The model under review builds one solid part; all positions refer to its coordinate system, in mm. A direction names the side the tool comes from. Round coordinates to 2 decimals unless told otherwise and drop trailing zeros. Order: outer loops, then holes, each group sorted by start corner. A loop starts at its lowest first (then second) coordinate and runs counter-clockwise, first axis right, second up.
1) Machinability: for faces 1 (the face through (-43, -12, -63)), 2 (the face through (27.5, 0, -7)), 3 (the face through (24.49, -20.6, 29.58)), 4 (the face through (24.54, 20.54, 29.58)), which of the approach directions +Z, -Z, +X, -X, +Y, -Y give a long, thin tool a straight path to every point of the face, cutting with its end or side? Answer none if there is none.
2) Consider section B-B (z = -100.25). Give the boundary of the cut face in (x, y), then the cut area to 3 significant figures.
3) Consider section D-D (x = 0). Give the boundary of the cut face in (y, z), then the cut area to 3 significant figures.
4) Mouldability with a two-part tool opening along Y and no side actions: class faces 5 (the face through (18.989, -22.576, 30.42)), 6 (the face through (16.04, 27.69, 29.58)), 7 (the face through (-38.7, -4.4, -3)) as pulls with the +Y half, pulls with the -Y half, needs draft (parallel to the pull), parting line crosses it, or undercut.
5) Consider section C-C (y = 0). Give the boundary of the cut face in (x, z).
6) To check wall thickness, follow L1, parallel to Y at x = 0, z = 59.1; L2, parallel to Y at x = 0, z = -78.25; L3, parallel to Z at x = 40, y = -11.4. State the ranges of each line that lie inside material, in increasing order.
7) Consider section A-A (x = -44.75). Give the boundary of the cut face in (y, z), then the cut area to 3 significant figures.
8) Clearance check with flat-ended pins moving along their axes: P1, Ø8, axis at y = 0, z = -6, coming from the +X side; P2, Ø2, axis at x = 34.5, y = -29.5, coming from the +Z side; P3, Ø0.5, axis at x = 42.5, y = -11.5, coming from the +Z side. State where each tip first meets the part, or that it passes through.
from build123d import *

# Parameters (mm, degrees)
CROQUIS1_R              = 32
SALIENTE_EXTRUIR1_DEPTH = 60
CROQUIS2_R              = 24.5
CORTAR_EXTRUIR1_DEPTH   = 2.5
CROQUIS3_W              = 5
CROQUIS3_H              = 5
CORTAR_EXTRUIR2_DEPTH   = 61
MATRIZC1_COUNT          = 18
CROQUIS4_R              = 26.25
SALIENTE_EXTRUIR2_DEPTH = 87.8
CROQUIS5_R              = 22.75
CORTAR_EXTRUIR3_DEPTH   = 37
SALIENTE_EXTRUIR3_REACH = 149.8
CROQUIS6_W              = 2.5
CROQUIS6_H              = 16
CROQUIS7_W              = 78
CROQUIS7_H              = 70
SALIENTE_EXTRUIR4_DEPTH = 61
CROQUIS8_W              = 10
CROQUIS8_H              = 1
SALIENTE_EXTRUIR5_DEPTH = 11.5
CROQUIS9_W              = 10
CROQUIS9_H              = 13
SALIENTE_EXTRUIR6_DEPTH = 1
CROQUIS10_W             = 11
CROQUIS10_H             = 10
SALIENTE_EXTRUIR7_DEPTH = 1
SALIENTE_EXTRUIR8_DEPTH = 1
CROQUIS12_R             = 2.5
CORTAR_EXTRUIR4_DEPTH   = 29
CROQUIS13_R             = 2.5
CORTAR_EXTRUIR5_DEPTH   = 1
CROQUIS14_R             = 2.5
CORTAR_EXTRUIR6_DEPTH   = 1
CROQUIS15_R             = 2.5
CORTAR_EXTRUIR7_DEPTH   = 1
CROQUIS16_R             = 3.5
SALIENTE_EXTRUIR9_DEPTH = 10


with BuildPart() as part:
    # Croquis1 → Saliente-Extruir1 (new body)
    with BuildSketch(Plane.XY):
        Circle(CROQUIS1_R)
    extrude(amount=SALIENTE_EXTRUIR1_DEPTH)

    # Croquis2 → Cortar-Extruir1 (cut)
    with BuildSketch(Plane.XY.offset(60)):
        Circle(CROQUIS2_R)
    extrude(amount=-CORTAR_EXTRUIR1_DEPTH, mode=Mode.SUBTRACT)

    # Croquis3 → Cortar-Extruir2 (cut, through all)
    with BuildSketch(Plane.XY.offset(60)):
        with Locations((0, 32)):
            Rectangle(CROQUIS3_W, CROQUIS3_H)
    cortar_extruir2 = extrude(amount=-CORTAR_EXTRUIR2_DEPTH, mode=Mode.SUBTRACT)

    # MatrizC1: Cortar-Extruir2 ×18 about axis
    matrizc1_axis = Axis((0, 0, 0), (0, 0, 1))
    for i in range(1, MATRIZC1_COUNT):
        add(cortar_extruir2.rotate(matrizc1_axis, i * 360 / MATRIZC1_COUNT), mode=Mode.SUBTRACT)

    # Croquis4 → Saliente-Extruir2 (add)
    with BuildSketch(Plane(origin=(0, 0, 0), x_dir=(-1, 0, 0), z_dir=(0, 0, -1))):
        Circle(CROQUIS4_R)
    extrude(amount=SALIENTE_EXTRUIR2_DEPTH)

    # Croquis5 → Cortar-Extruir3 (cut)
    with BuildSketch(Plane(origin=(0, 0, -87.8), x_dir=(-1, 0, 0), z_dir=(0, 0, -1))):
        Circle(CROQUIS5_R)
    extrude(amount=-CORTAR_EXTRUIR3_DEPTH, mode=Mode.SUBTRACT)

    # Croquis6 → Saliente-Extruir3 (add, up to next)
    with BuildSketch(Plane(origin=(0, 0, -87.8), x_dir=(-1, 0, 0), z_dir=(0, 0, -1)), mode=Mode.PRIVATE) as saliente_extruir3_sk1:
        with Locations((-26.25, 0)):
            Rectangle(CROQUIS6_W, CROQUIS6_H)
    saliente_extruir3_tool1 = extrude(saliente_extruir3_sk1.sketch, amount=-SALIENTE_EXTRUIR3_REACH, mode=Mode.PRIVATE) - part.part
    add(saliente_extruir3_tool1.solids().sort_by_distance((26.25, 0, -87.8))[0])

    # Croquis7 → Saliente-Extruir4 (add)
    with BuildSketch(Plane(origin=(0, 0, -13), x_dir=(-1, 0, 0), z_dir=(0, 0, -1))):
        Rectangle(CROQUIS7_W, CROQUIS7_H)
    extrude(amount=SALIENTE_EXTRUIR4_DEPTH)

    # Croquis8 → Saliente-Extruir5 (add)
    with BuildSketch(Plane.ZY.offset(39)):
        with Locations((-64.8, -11.5)):
            Rectangle(CROQUIS8_W, CROQUIS8_H)
        with Locations((-8, -7.5)):
            Rectangle(CROQUIS8_W, CROQUIS8_H)
    extrude(amount=SALIENTE_EXTRUIR5_DEPTH)

    # Croquis9 → Saliente-Extruir6 (add)
    with BuildSketch(Plane.ZY.offset(39)):
        with Locations((-8, -1.5)):
            Rectangle(CROQUIS9_W, CROQUIS9_H)
    extrude(amount=-SALIENTE_EXTRUIR6_DEPTH)

    # Croquis10 → Saliente-Extruir7 (add)
    with BuildSketch(Plane(origin=(0, -11, 0), x_dir=(-1, 0, 0), z_dir=(0, -1, 0))):
        with Locations((-40.6, 8)):
            Rectangle(CROQUIS10_W, CROQUIS10_H)
    extrude(amount=SALIENTE_EXTRUIR7_DEPTH)

    # Croquis11 → Saliente-Extruir8 (add)
    with BuildSketch(Plane(origin=(0, -11, 0), x_dir=(-1, 0, 0), z_dir=(0, -1, 0))):
        Polygon((-39, 74), (-28, 74), (-28, 106), (-45.5, 106), (-45.5, 94.5), (-39, 94.5), align=None)
    extrude(amount=SALIENTE_EXTRUIR8_DEPTH)

    # Croquis12 → Cortar-Extruir4 (cut, through all)
    with BuildSketch(Plane(origin=(0, -7, 0), x_dir=(1, 0, 0), z_dir=(0, 1, 0))):
        with Locations((-44.75, 7.949105166)):
            Circle(CROQUIS12_R)
    extrude(amount=-CORTAR_EXTRUIR4_DEPTH, mode=Mode.SUBTRACT)

    # Croquis13 → Cortar-Extruir5 (cut)
    with BuildSketch(Plane(origin=(0, -11, 0), x_dir=(1, 0, 0), z_dir=(0, 1, 0))):
        with Locations((40.6, 7.978589127)):
            Circle(CROQUIS13_R)
    extrude(amount=-CORTAR_EXTRUIR5_DEPTH, mode=Mode.SUBTRACT)

    # Croquis14 → Cortar-Extruir6 (cut)
    with BuildSketch(Plane(origin=(0, -11, 0), x_dir=(1, 0, 0), z_dir=(0, 1, 0))):
        with Locations((-44.75, 65.049509944)):
            Circle(CROQUIS14_R)
    extrude(amount=-CORTAR_EXTRUIR6_DEPTH, mode=Mode.SUBTRACT)

    # Croquis15 → Cortar-Extruir7 (cut)
    with BuildSketch(Plane(origin=(0, -11, 0), x_dir=(1, 0, 0), z_dir=(0, 1, 0))):
        with Locations((40, 100.25)):
            Circle(CROQUIS15_R)
    extrude(amount=-CORTAR_EXTRUIR7_DEPTH, mode=Mode.SUBTRACT)

    # Croquis16 → Saliente-Extruir9 (add)
    with BuildSketch(Plane(origin=(0, -35, 0), x_dir=(-1, 0, 0), z_dir=(0, -1, 0))):
        with Locations((-26.5, 32)):
            Circle(CROQUIS16_R)
    extrude(amount=SALIENTE_EXTRUIR9_DEPTH)


solid = part.part
Answer below:
1. face 1: +Z, -Z, -X, -Y
1. face 2: +X, +Y, -Y
1. face 3: +Z, +X, -Y
1. face 4: +Z, +X, +Y
2. outline: (28, -12) - (37.5, -12) - (37.5, -11) - (28, -11) - close; (42.5, -12) - (45.5, -12) - (45.5, -11) - (42.5, -11) - close
2. area: 12.5 mm2
3. outline: (-35, -74) - (-26.25, -74) - (-26.25, -87.8) - (-22.75, -87.8) - (-22.75, -74) - (22.75, -74) - (22.75, -87.8) - (26.25, -87.8) - (26.25, -74) - (35, -74) - (35, -13) - (26.25, -13) - (26.25, 0) - (29.5, 0) - (29.5, 60) - (24.5, 60) - (24.5, 57.5) - (-24.5, 57.5) - (-24.5, 60) - (-29.5, 60) - (-29.5, 0) - (-26.25, 0) - (-26.25, -13) - (-35, -13) - close
3. area: 8,470 mm2
4. face 5: undercut
4. face 6: pulls with the +Y half
4. face 7: needs draft
5. outline: (-39, -74) - (-26.25, -74) - (-26.25, -87.8) - (-22.75, -87.8) - (-22.75, -74) - (22.75, -74) - (22.75, -87.8) - (27.5, -87.8) - (27.5, -74) - (39, -74) - (39, -13) - (27.5, -13) - (27.5, 0) - (32, 0) - (32, 60) - (24.5, 60) - (24.5, 57.5) - (-24.5, 57.5) - (-24.5, 60) - (-32, 60) - (-32, 0) - (-26.25, 0) - (-26.25, -13) - (-38, -13) - (-38, -3) - (-39, -3) - close
6. L1: y = -29.5 to -24.5, 24.5 to 29.5
6. L2: y = -26.25 to -22.75, 22.75 to 26.25
6. L3: z = -106 to -102.75, -97.75 to -94.5, -13 to -10.41, -5.55 to -3
7. outline: (-12, -69.8) - (-11, -69.8) - (-11, -67.55) - (-12, -67.55) - close; (-12, -62.55) - (-11, -62.55) - (-11, -59.8) - (-12, -59.8) - close; (-8, -13) - (-7, -13) - (-7, -10.45) - (-8, -10.45) - close; (-8, -5.45) - (-7, -5.45) - (-7, -3) - (-8, -3) - close
7. area: 10.0 mm2
8. P1: stops at x = 27.5
8. P2: stops at z = -13
8. P3: stops at z = -3
